Input: part model. Units: mm. Frame: model coordinates. Face numbers are marked on the shaded views. A direction names the side the tool comes from. Coordinates: 2 decimals unless noted, no trailing zeros. Order: outer loops, then holes, each group sorted by start corner. A loop starts at its lowest first (then second) coordinate and runs counter-clockwise, first axis right, second up. Notation, with made-up numbers: (47, 3) -> (95, 3) arc R20 cw to (95, 9) -> close; hole circle Ø7 at (-1, 57). An arc over 180 degrees is marked (long way). Use one line per item in the form item = value. Start each with the question number.
1) Pin query (flat end, axial travel): pin 1 (1.2 mm diameter, centred on y = 2, z = 1.5, fed in from -X); pin 2 (2 mm diameter, centred on x = 16.5, z = 2.5, fed in from -Y). Return the tip coordinate at first contact, or that it passes through.
2) Access query for the marked faces 1, 2, 3 and 4. Directions: +Z, -Z, +X, -X, +Y, -Y. A direction counts if a zero-diameter tool reaches every point of the face in a straight line with its end or side. Return the directions, or none.
3) Ray query, line 1 along X through (y, z) = (8.5, 0.35); line 2 along Y through (x, z) = (31.5, 1.5); line 3 along X through (y, z) = (3.5, 0.85). Return the intervals inside material, ascending.
4) Section query B-B on y = 9.5. Output: boundary loops of the cut face in (x, z).
5) Draft query along X for the marked faces 5, 6 and 7. Return one class per face: pulls with the +X half, pulls with the -X half, needs draft (parallel to the pull), parting line crosses it, or undercut.
6) Section query C-C on z = 2.1. Output: boundary loops of the cut face in (x, y), then the cut area to 3 significant figures.
7) Section query A-A on x = 30. Output: boundary loops of the cut face in (y, z).
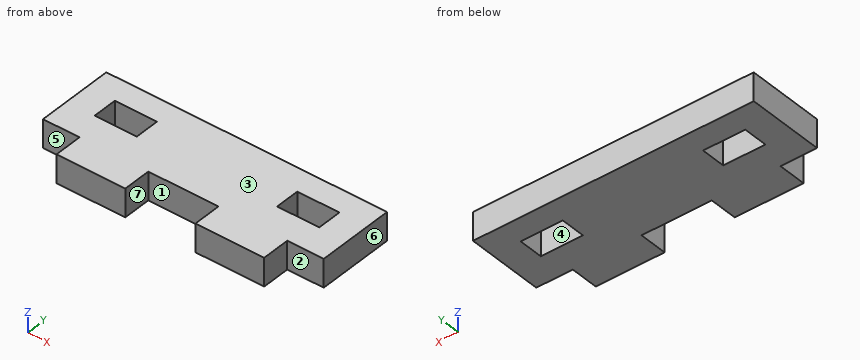
from build123d import *

# Parameters (mm, degrees)
AUFSATZ_LINEAR_AUSTRAGEN1_DEPTH = 4
SCHNITT_LINEAR_AUSTRAGEN1_REACH = 6
SKIZZE3_W                       = 2.7
SKIZZE3_H                       = 4
SKIZZE3_W_2                     = 10
SCHNITT_LINEAR_AUSTRAGEN2_REACH = 6
SKIZZE4_W                       = 6
SKIZZE4_H                       = 3.5


with BuildPart() as part:
    # Skizze2 → Aufsatz-Linear austragen1 (new body)
    with BuildSketch(Plane.XY):
        Polygon((0, 0), (0, 4), (-2.5, 4), (-2.5, 15), (37.5, 15), (37.5, 4), (35, 4), (35, 0), align=None)
    extrude(amount=AUFSATZ_LINEAR_AUSTRAGEN1_DEPTH)

    # Skizze3 → Schnitt-Linear austragen1 (cut, up to next)
    with BuildSketch(Plane.XY.offset(4), mode=Mode.PRIVATE) as schnitt_linear_austragen1_sk1:
        with Locations((1.35, 2)):
            Rectangle(SKIZZE3_W, SKIZZE3_H)
    schnitt_linear_austragen1_tool1 = extrude(schnitt_linear_austragen1_sk1.sketch, amount=-SCHNITT_LINEAR_AUSTRAGEN1_REACH, mode=Mode.PRIVATE) & part.part
    add(schnitt_linear_austragen1_tool1.solids().sort_by_distance((1.35, 2, 4))[0], mode=Mode.SUBTRACT)
    # Skizze3 → Schnitt-Linear austragen1 (cut, up to next)
    with BuildSketch(Plane.XY.offset(4), mode=Mode.PRIVATE) as schnitt_linear_austragen1_sk2:
        with Locations((17.5, 2)):
            Rectangle(SKIZZE3_W_2, SKIZZE3_H)
    schnitt_linear_austragen1_tool2 = extrude(schnitt_linear_austragen1_sk2.sketch, amount=-SCHNITT_LINEAR_AUSTRAGEN1_REACH, mode=Mode.PRIVATE) & part.part
    add(schnitt_linear_austragen1_tool2.solids().sort_by_distance((17.5, 2, 4))[0], mode=Mode.SUBTRACT)
    # Skizze3 → Schnitt-Linear austragen1 (cut, up to next)
    with BuildSketch(Plane.XY.offset(4), mode=Mode.PRIVATE) as schnitt_linear_austragen1_sk3:
        with Locations((33.65, 2)):
            Rectangle(SKIZZE3_W, SKIZZE3_H)
    schnitt_linear_austragen1_tool3 = extrude(schnitt_linear_austragen1_sk3.sketch, amount=-SCHNITT_LINEAR_AUSTRAGEN1_REACH, mode=Mode.PRIVATE) & part.part
    add(schnitt_linear_austragen1_tool3.solids().sort_by_distance((33.65, 2, 4))[0], mode=Mode.SUBTRACT)

    # Skizze4 → Schnitt-Linear austragen2 (cut, up to next)
    with BuildSketch(Plane.XY.offset(4), mode=Mode.PRIVATE) as schnitt_linear_austragen2_sk1:
        with Locations((4.5, 9.85)):
            Rectangle(SKIZZE4_W, SKIZZE4_H)
    schnitt_linear_austragen2_tool1 = extrude(schnitt_linear_austragen2_sk1.sketch, amount=-SCHNITT_LINEAR_AUSTRAGEN2_REACH, mode=Mode.PRIVATE) & part.part
    add(schnitt_linear_austragen2_tool1.solids().sort_by_distance((4.5, 9.85, 4))[0], mode=Mode.SUBTRACT)
    # Skizze4 → Schnitt-Linear austragen2 (cut, up to next)
    with BuildSketch(Plane.XY.offset(4), mode=Mode.PRIVATE) as schnitt_linear_austragen2_sk2:
        with Locations((30.5, 9.85)):
            Rectangle(SKIZZE4_W, SKIZZE4_H)
    schnitt_linear_austragen2_tool2 = extrude(schnitt_linear_austragen2_sk2.sketch, amount=-SCHNITT_LINEAR_AUSTRAGEN2_REACH, mode=Mode.PRIVATE) & part.part
    add(schnitt_linear_austragen2_tool2.solids().sort_by_distance((30.5, 9.85, 4))[0], mode=Mode.SUBTRACT)


solid = part.part
Answers below:
q1.pin_1 = 2.7
q1.pin_2 = 4
q2.face_1 = +Z, -Z, -Y
q2.face_2 = +Z, -Z, +X, -Y
q2.face_3 = +Z, +X, -X, +Y, -Y
q2.face_4 = +Z, -Z
q3.line_1 = -2.5 to 1.5, 7.5 to 27.5, 33.5 to 37.5
q3.line_2 = 0 to 8.1, 11.6 to 15
q3.line_3 = 2.7 to 12.5, 22.5 to 32.3
q4.outline = (-2.5, 0) -> (1.5, 0) -> (1.5, 4) -> (-2.5, 4) -> close; (7.5, 0) -> (27.5, 0) -> (27.5, 4) -> (7.5, 4) -> close; (33.5, 0) -> (37.5, 0) -> (37.5, 4) -> (33.5, 4) -> close
q5.face_5 = needs draft
q5.face_6 = pulls with the +X half
q5.face_7 = undercut
q6.outline = (-2.5, 4) -> (2.7, 4) -> (2.7, 0) -> (12.5, 0) -> (12.5, 4) -> (22.5, 4) -> (22.5, 0) -> (32.3, 0) -> (32.3, 4) -> (37.5, 4) -> (37.5, 15) -> (-2.5, 15) -> close; hole (1.5, 8.1) -> (7.5, 8.1) -> (7.5, 11.6) -> (1.5, 11.6) -> close; hole (27.5, 8.1) -> (33.5, 8.1) -> (33.5, 11.6) -> (27.5, 11.6) -> close
q6.area = 476 mm^2
q7.outline = (0, 0) -> (8.1, 0) -> (8.1, 4) -> (0, 4) -> close; (11.6, 0) -> (15, 0) -> (15, 4) -> (11.6, 4) -> close
